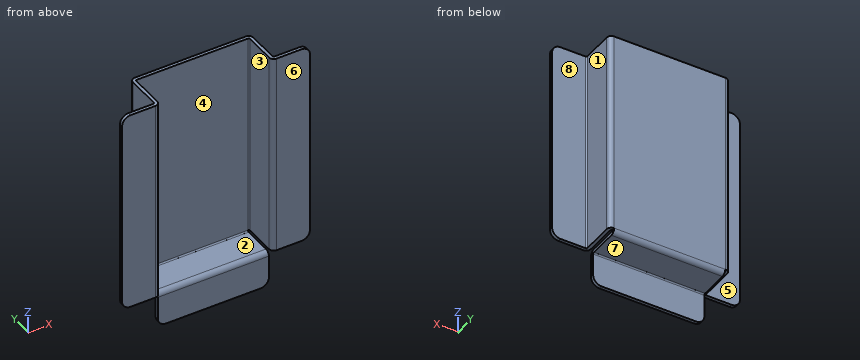
from build123d import *

# Parameters (mm, degrees)
SKETCH3_W                    = 66.802
SKETCH3_H                    = 120
BASE_FLANGE1_DEPTH           = 1.99
EDGE_FLANGE1_STRIP_W         = 9.4332
EDGE_FLANGE1_STRIP_H         = 1.99
EDGE_FLANGE1_STRIP_CUT_DEPTH = 120
EDGE_FLANGE1_DEPTH           = 120
EDGE_FLANGE2_STRIP_W         = 9.4332
EDGE_FLANGE2_STRIP_H         = 1.99
EDGE_FLANGE2_STRIP_CUT_DEPTH = 120
EDGE_FLANGE2_DEPTH           = 120
EDGE_FLANGE3_STRIP_W         = 9.4332
EDGE_FLANGE3_STRIP_H         = 1.99
EDGE_FLANGE3_STRIP_CUT_DEPTH = 120
EDGE_FLANGE3_DEPTH           = 120
EDGE_FLANGE4_STRIP_W         = 9.4332
EDGE_FLANGE4_STRIP_H         = 1.99
EDGE_FLANGE4_STRIP_CUT_DEPTH = 120
EDGE_FLANGE4_DEPTH           = 120
EDGE_FLANGE6_DEPTH           = 65.3288
EDGE_FLANGE7_STRIP_W         = 9.4332
EDGE_FLANGE7_STRIP_H         = 1.99
EDGE_FLANGE7_STRIP_CUT_DEPTH = 65.3288
EDGE_FLANGE7_DEPTH           = 65.3288
FILLET1_R                    = 5


# Sheet-metal steps are written as plain solids
with BuildPart() as part:
    # Sketch3 → Base-Flange1 (new body)
    with BuildSketch(Plane(origin=(0, 0, 0), x_dir=(1, 0, 0), z_dir=(0, 1, 0))):
        Rectangle(SKETCH3_W, SKETCH3_H)
    extrude(amount=-BASE_FLANGE1_DEPTH)

    # Edge-Flange1 strip (across the edge) → Edge-Flange1 strip cut (cut)
    with BuildSketch(Plane(origin=(33.401, -1.99, -60), x_dir=(-1, 0, 0), z_dir=(0, 0, 1))):
        with Locations((-3.98, -0.995)):
            Rectangle(EDGE_FLANGE1_STRIP_W, EDGE_FLANGE1_STRIP_H)
    extrude(amount=EDGE_FLANGE1_STRIP_CUT_DEPTH, mode=Mode.SUBTRACT)

    # Edge-Flange1 section (across the edge) → Edge-Flange1 (add)
    with BuildSketch(Plane(origin=(33.401, -1.99, -60), x_dir=(-1, 0, 0), z_dir=(0, 0, 1))):
        with BuildLine():
            Line((-1.99, 0.7366), (-1.99, 21.71))
            Line((-1.99, 21.71), (0, 21.71))
            Line((0, 21.71), (0, 0.7366))
            ThreePointArc((0, 0.7366), (0.215745145, 0.215745145), (0.7366, 0))
            Line((0.7366, 0), (0.7366, -1.99))
            ThreePointArc((0.7366, -1.99), (-1.19139735, -1.19139735), (-1.99, 0.7366))
        make_face()
    extrude(amount=EDGE_FLANGE1_DEPTH)

    # Edge-Flange2 strip (across the edge) → Edge-Flange2 strip cut (cut)
    with BuildSketch(Plane(origin=(-33.401, -1.99, 60), x_dir=(1, 0, 0), z_dir=(0, 0, -1))):
        with Locations((-3.98, -0.995)):
            Rectangle(EDGE_FLANGE2_STRIP_W, EDGE_FLANGE2_STRIP_H)
    extrude(amount=EDGE_FLANGE2_STRIP_CUT_DEPTH, mode=Mode.SUBTRACT)

    # Edge-Flange2 section (across the edge) → Edge-Flange2 (add)
    with BuildSketch(Plane(origin=(-33.401, -1.99, 60), x_dir=(1, 0, 0), z_dir=(0, 0, -1))):
        with BuildLine():
            Line((-1.99, 0.7366), (-1.99, 23.41))
            Line((-1.99, 23.41), (0, 23.41))
            Line((0, 23.41), (0, 0.7366))
            ThreePointArc((0, 0.7366), (0.215745145, 0.215745145), (0.7366, 0))
            Line((0.7366, 0), (0.7366, -1.99))
            ThreePointArc((0.7366, -1.99), (-1.19139735, -1.19139735), (-1.99, 0.7366))
        make_face()
    extrude(amount=EDGE_FLANGE2_DEPTH)

    # Edge-Flange3 strip (across the edge) → Edge-Flange3 strip cut (cut)
    with BuildSketch(Plane(origin=(35.391, -23.7, 60), x_dir=(0, 1, 0), z_dir=(0, 0, -1))):
        with Locations((-1.99, -0.995)):
            Rectangle(EDGE_FLANGE3_STRIP_W, EDGE_FLANGE3_STRIP_H)
    extrude(amount=EDGE_FLANGE3_STRIP_CUT_DEPTH, mode=Mode.SUBTRACT)

    # Edge-Flange3 section (across the edge) → Edge-Flange3 (add)
    with BuildSketch(Plane(origin=(35.391, -23.7, 60), x_dir=(0, 1, 0), z_dir=(0, 0, -1))):
        with BuildLine():
            Line((0, 0.7366), (0, 20.362))
            Line((0, 20.362), (1.99, 20.362))
            Line((1.99, 20.362), (1.99, 0.7366))
            ThreePointArc((1.99, 0.7366), (2.205745145, 0.215745145), (2.7266, 0))
            Line((2.7266, 0), (2.7266, -1.99))
            ThreePointArc((2.7266, -1.99), (0.79860265, -1.19139735), (0, 0.7366))
        make_face()
    extrude(amount=EDGE_FLANGE3_DEPTH)

    # Edge-Flange4 strip (across the edge) → Edge-Flange4 strip cut (cut)
    with BuildSketch(Plane(origin=(-35.391, -25.4, -60), x_dir=(0, 1, 0), z_dir=(0, 0, 1))):
        with Locations((-1.99, -0.995)):
            Rectangle(EDGE_FLANGE4_STRIP_W, EDGE_FLANGE4_STRIP_H)
    extrude(amount=EDGE_FLANGE4_STRIP_CUT_DEPTH, mode=Mode.SUBTRACT)

    # Edge-Flange4 section (across the edge) → Edge-Flange4 (add)
    with BuildSketch(Plane(origin=(-35.391, -25.4, -60), x_dir=(0, 1, 0), z_dir=(0, 0, 1))):
        with BuildLine():
            Line((0, 0.7366), (0, 20.362))
            Line((0, 20.362), (1.99, 20.362))
            Line((1.99, 20.362), (1.99, 0.7366))
            ThreePointArc((1.99, 0.7366), (2.205745145, 0.215745145), (2.7266, 0))
            Line((2.7266, 0), (2.7266, -1.99))
            ThreePointArc((2.7266, -1.99), (0.79860265, -1.19139735), (0, 0.7366))
        make_face()
    extrude(amount=EDGE_FLANGE4_DEPTH)

    # Edge-Flange6 section (across the edge) → Edge-Flange6 (add)
    with BuildSketch(Plane(origin=(-32.6644, -1.99, -60.7366), x_dir=(0, 0, 1), z_dir=(1, 0, 0))):
        with BuildLine():
            Line((-1.99, 0.7366), (-1.99, 17.99))
            Line((-1.99, 17.99), (0, 17.99))
            Line((0, 17.99), (0, 0.7366))
            ThreePointArc((0, 0.7366), (0.215745145, 0.215745145), (0.7366, 0))
            Line((0.7366, 0), (0.7366, -1.99))
            ThreePointArc((0.7366, -1.99), (-1.19139735, -1.19139735), (-1.99, 0.7366))
        make_face()
    extrude(amount=EDGE_FLANGE6_DEPTH)

    # Edge-Flange7 strip (across the edge) → Edge-Flange7 strip cut (cut)
    with BuildSketch(Plane(origin=(32.6644, -19.98, -62.7266), x_dir=(0, 1, 0), z_dir=(-1, 0, 0))):
        with Locations((-3.98, -0.995)):
            Rectangle(EDGE_FLANGE7_STRIP_W, EDGE_FLANGE7_STRIP_H)
    extrude(amount=EDGE_FLANGE7_STRIP_CUT_DEPTH, mode=Mode.SUBTRACT)

    # Edge-Flange7 section (across the edge) → Edge-Flange7 (add)
    with BuildSketch(Plane(origin=(32.6644, -19.98, -62.7266), x_dir=(0, 1, 0), z_dir=(-1, 0, 0))):
        with BuildLine():
            Line((-1.99, 0.7366), (-1.99, 19.01))
            Line((-1.99, 19.01), (0, 19.01))
            Line((0, 19.01), (0, 0.7366))
            ThreePointArc((0, 0.7366), (0.215745145, 0.215745145), (0.7366, 0))
            Line((0.7366, 0), (0.7366, -1.99))
            ThreePointArc((0.7366, -1.99), (-1.19139735, -1.19139735), (-1.99, 0.7366))
        make_face()
    extrude(amount=EDGE_FLANGE7_DEPTH)

    # Fillet1
    fillet1_edges = [part.edges().sort_by_distance(p)[0] for p in [
        (55.753, -22.705, 60),
        (55.753, -22.705, -60),
        (-55.753, -24.405, -60),
        (-55.753, -24.405, 60),
        (32.6644, -20.975, -81.7366),
        (-32.6644, -20.975, -81.7366),
    ]]
    fillet(fillet1_edges, radius=FILLET1_R)


solid = part.part
Can you work these out from the model? Positions are in its coordinate system, mm. Face numbers are marked on the shaded views. A direction names the side the tool comes from. Coordinates: 2 decimals unless noted, no trailing zeros. Write each loop counter-clockwise with the first axis right and the second up, starting at its lowest first coordinate (ties: lowest second). Pieces come first, ordered by that corner, then holes.
Q1. Which directions (+Z, -Z, +X, -X, +Y, -Y) give clear straight access to the entire face, cutting with the end or side of a thin tool? Please do the marked faces 5, 6, 7 and 8.
Results found:
face 5: +Z, -Z, -X, +Y
face 6: +Z, -Z, +X, -Y
face 7: -Z, +X, -X, +Y
face 8: +Z, -Z, +X, +Y
Q2. Please list where these lines run through material, in increasing order: L1, parallel to X at y = -19, z = -40; L2, parallel to Y at x = -8.5, z = -41; L3, parallel to Y at x = 37, z = 11.
Results found:
L1: x = -35.39 to -33.4, 33.4 to 35.39
L2: y = -1.99 to 0
L3: y = -23.7 to -21.71
Q3. Imagine slicing it at B-B, the plane x = 18. List the corners of the cut face in (y, z) for me.
Results found:
outline: (-21.97, -81.74) - (-19.98, -81.74) - (-19.98, -63.46) arc R0.74 cw to (-19.24, -62.73) - (-2.73, -62.73) arc R2.73 ccw to (0, -60) - (0, 60) - (-1.99, 60) - (-1.99, -60) arc R0.74 cw to (-2.73, -60.74) - (-19.24, -60.74) arc R2.73 ccw to (-21.97, -63.46) - close
Q4. Imagine slicing it at C-C, the plane z = -53. List the corners of the cut face in (x, y) for me.
Results found:
outline: (-55.75, -25.4) - (-36.13, -25.4) arc R2.73 ccw to (-33.4, -22.67) - (-33.4, -2.73) arc R0.74 cw to (-32.66, -1.99) - (32.66, -1.99) arc R0.74 cw to (33.4, -2.73) - (33.4, -20.97) arc R2.73 ccw to (36.13, -23.7) - (55.75, -23.7) - (55.75, -21.71) - (36.13, -21.71) arc R0.74 cw to (35.39, -20.97) - (35.39, -2.73) arc R2.73 ccw to (32.66, 0) - (-32.66, 0) arc R2.73 ccw to (-35.39, -2.73) - (-35.39, -22.67) arc R0.74 cw to (-36.13, -23.41) - (-55.75, -23.41) - close
Q5. Imagine slicing it at D-D, the plane x = -40.5. List the corners of the cut face in (y, z) for me.
Results found:
outline: (-25.4, -60) - (-23.41, -60) - (-23.41, 60) - (-25.4, 60) - close
Q6. For P1, Ø12, axis at y = -15, z = -39, coming from the -X side; P2, Ø1, axis at y = -5.5, z = -63, coming from the -X side; P3, Ø2, axis at x = -2, z = -60.5, coming from the -Y side, each with a flat end and sliding along its axis, tell me the tip position at first contact or that it passes through.
Results found:
P1: stops at x = -35.39
P2: stops at x = -32.66
P3: stops at y = -21.14
Q7. Imagine slicing it at A-A, the plane y = -14.5. List the corners of the cut face in (x, z) for me, plus the area to 3 significant figures.
Results found:
outline: (-35.39, -60) - (-33.4, -60) - (-33.4, 60) - (-35.39, 60) - close; (-32.66, -62.73) - (32.66, -62.73) - (32.66, -60.74) - (-32.66, -60.74) - close; (33.4, -60) - (35.39, -60) - (35.39, 60) - (33.4, 60) - close
area: 608 mm2
Q8. If we mould it in two halves opening along X, with no side actions, what happens to the marked faces 1, 2, 3 and 4? For each: +X half, -X half, draft (parallel to the pull), parting line (faces both ways), or undercut.
Results found:
face 1: +X half
face 2: draft
face 3: undercut
face 4: undercut
